Part model, mm, in its own coordinate system. Give positions to 0.01 mm unless a question says otherwise; leave off trailing zeros. Answer as CSV lines item,"result". Start each with the question number.
Item 1: Wall check: L1, parallel to Y at x = 33, z = 515; L2, parallel to X at y = -1, z = 768; L3, parallel to X at y = -3, z = 987. Give the ranges that are in metal, low to high. Write a range as from..to.
Item 2: Pin check, flat tips, straight feed: pin 1 (6 mm diameter, centred on x = 19.64, y = -15.81, fed in from +Z); pin 2 (1.5 mm diameter, centred on x = 19.5, z = 729, fed in from +Y); pin 3 (1 mm diameter, centred on x = 18.5, z = 854.5, fed in from -Y). Stop position of each tip, or through.
Item 3: Band-saw the part on A-A, the plane z = 664.5. Count the separate pieces of the cut face and the enclosed holes in it, then the cut area to 3 significant figures.
from build123d import *

# Parameters (mm, degrees)
F0_R     = 4
F0_R_2   = 3.25
F1_DEPTH = 1200


with BuildPart() as f1:
    # F0 (on Top) → F1 (new body)
    with BuildSketch(Plane.XY):
        with BuildLine():
            Line((15.640583, 4.190956), (-0.359417, 4.190956))
            Line((-0.359417, 4.190956), (-0.359417, -11.809044))
            Line((-0.359417, -11.809044), (3.640583, -11.809044))
            Line((3.640583, -11.809044), (3.640583, -8.809044))
            Line((3.640583, -8.809044), (10.640583, -8.809044))
            ThreePointArc((10.640583, -8.809044), (13.540078, -15.809044), (10.640583, -22.809044))
            Line((10.640583, -22.809044), (3.640583, -22.809044))
            Line((3.640583, -22.809044), (3.640583, -19.809044))
            Line((3.640583, -19.809044), (-0.359417, -19.809044))
            Line((-0.359417, -19.809044), (-0.359417, -35.809044))
            Line((-0.359417, -35.809044), (15.640583, -35.809044))
            Line((15.640583, -35.809044), (15.640583, -31.809044))
            Line((15.640583, -31.809044), (12.640583, -31.809044))
            Line((12.640583, -31.809044), (12.640583, -24.809044))
            ThreePointArc((12.640583, -24.809044), (19.640583, -21.909549), (26.640583, -24.809044))
            Line((26.640583, -24.809044), (26.640583, -31.809044))
            Line((26.640583, -31.809044), (23.640583, -31.809044))
            Line((23.640583, -31.809044), (23.640583, -35.809044))
            Line((23.640583, -35.809044), (39.640583, -35.809044))
            Line((39.640583, -35.809044), (39.640583, -19.809044))
            Line((39.640583, -19.809044), (35.640583, -19.809044))
            Line((35.640583, -19.809044), (35.640583, -22.809044))
            Line((35.640583, -22.809044), (28.640583, -22.809044))
            ThreePointArc((28.640583, -22.809044), (25.741088, -15.809044), (28.640583, -8.809044))
            Line((28.640583, -8.809044), (35.640583, -8.809044))
            Line((35.640583, -8.809044), (35.640583, -11.809044))
            Line((35.640583, -11.809044), (39.640583, -11.809044))
            Line((39.640583, -11.809044), (39.640583, 4.190956))
            Line((39.640583, 4.190956), (23.640583, 4.190956))
            Line((23.640583, 4.190956), (23.640583, 0.190956))
            Line((23.640583, 0.190956), (26.640583, 0.190956))
            Line((26.640583, 0.190956), (26.640583, -6.809044))
            ThreePointArc((26.640583, -6.809044), (19.640583, -9.708539), (12.640583, -6.809044))
            Line((12.640583, -6.809044), (12.640583, 0.190956))
            Line((12.640583, 0.190956), (15.640583, 0.190956))
            Line((15.640583, 0.190956), (15.640583, 4.190956))
        make_face()
        with Locations((5.650991, -29.798636)):
            Circle(F0_R, mode=Mode.SUBTRACT)
        with Locations((33.630175, -29.798636)):
            Circle(F0_R, mode=Mode.SUBTRACT)
        with Locations((5.650991, -1.819451)):
            Circle(F0_R, mode=Mode.SUBTRACT)
        with Locations((19.640583, -15.809044)):
            Circle(F0_R_2, mode=Mode.SUBTRACT)
        with Locations((33.630175, -1.819451)):
            Circle(F0_R, mode=Mode.SUBTRACT)
    extrude(amount=F1_DEPTH)


solid = f1.part
Output:
1,L1,"-35.81..-33.75, -25.85..-22.81, -8.81..-5.77, 2.13..4.19"
1,L2,"-0.36..1.74, 9.57..12.64, 26.64..29.72, 37.55..39.64"
1,L3,"-0.36..1.83, 9.47..12.64, 26.64..29.81, 37.45..39.64"
2,pin 1,"through"
2,pin 2,"y = -9.67"
2,pin 3,"y = -22.05"
3,separate pieces,"1"
3,enclosed holes,"5"
3,area,"734 mm²"
